Read the model definition and answer for the solid it produces. Units are mm, in the model's axes. Face numbers are marked on the shaded views. Coordinates: 2 decimals unless noted, no trailing zeros. Write each loop counter-clockwise with the first axis right and the second up, starting at its lowest first coordinate (ties: lowest second). Pieces come first, ordered by that corner, then holes.
(1) Straight lines are drawn through the part: line 1 along X through (y, z) = (0, -6.25); line 2 along Y through (x, z) = (0, 10.25). For each, find the intervals that lie inside material, in ascending order.
(2) The part is cut by section A-A, the plane x = 0. Determine the outline of the cut face in (y, z).
(3) The part is cut by section C-C, the plane z = 16.5. Determine the outline of the cut face in (x, y), and give its area (3 significant figures).
(4) Determine the mould class of the marked faces 1, 2 and 3 for opening direction X: pulls with the +X half, pulls with the -X half, needs draft (parallel to the pull), parting line crosses it, or undercut.
(5) Given pin 1 (5.5 mm diameter, centred on x = 0, y = 0, fed in from +Z); pin 2 (2 mm diameter, centred on y = -2.5, z = 9, fed in from +X); pin 3 (1.5 mm diameter, centred on x = 3, z = 17, fed in from +Y); pin 4 (1 mm diameter, centred on y = -1.5, z = 11.5, fed in from -X), each flat-ended and moving along its own axis, determine where each tip first touches the part or whether it passes through.
(6) The part is cut by section D-D, the plane z = -2. Determine the outline of the cut face in (x, y).
```python
from build123d import *

# Parameters (mm, degrees)
F0_R     = 6
F0_R_2   = 4
F1_DEPTH = 4
F2_DEPTH = 4
F3_R     = 6
F3_R_2   = 4.5
F4_DEPTH = 20
F5_R     = 6
F5_R_2   = 4.45
F6_DEPTH = 15
F7_SIZE  = 0.4
F8_R     = 1


with BuildPart() as f1:
    # F0 (on Top) → F1 (new body)
    with BuildSketch(Plane.XY):
        Circle(F0_R)
        Circle(F0_R_2, mode=Mode.SUBTRACT)
    extrude(amount=F1_DEPTH)

    # F0 (on Top) → F2 (join)
    with BuildSketch(Plane.XY):
        Circle(F0_R)
        Circle(F0_R_2, mode=Mode.SUBTRACT)
    extrude(amount=F2_DEPTH)

    # F3 (on face) → F4 (join)
    with BuildSketch(Plane.XY.offset(4)):
        Circle(F3_R)
        Circle(F3_R_2, mode=Mode.SUBTRACT)
    extrude(amount=F4_DEPTH)

    # F5 (on face) → F6 (join)
    with BuildSketch(Plane(origin=(0, 0, 0), x_dir=(1, 0, 0), z_dir=(0, 0, -1))):
        Circle(F5_R)
        Circle(F5_R_2, mode=Mode.SUBTRACT)
    extrude(amount=F6_DEPTH)

    # F7
    f7_edges = [f1.edges().sort_by_distance(p)[0] for p in [
        (-4.45, 0, -15),
        (-4.5, 0, 24),
    ]]
    chamfer(f7_edges, length=F7_SIZE)

    # F8
    f8_edges = [f1.edges().sort_by_distance(p)[0] for p in [
        (-6, 0, 24),
        (-6, 0, -15),
    ]]
    fillet(f8_edges, radius=F8_R)


solid = f1.part
```
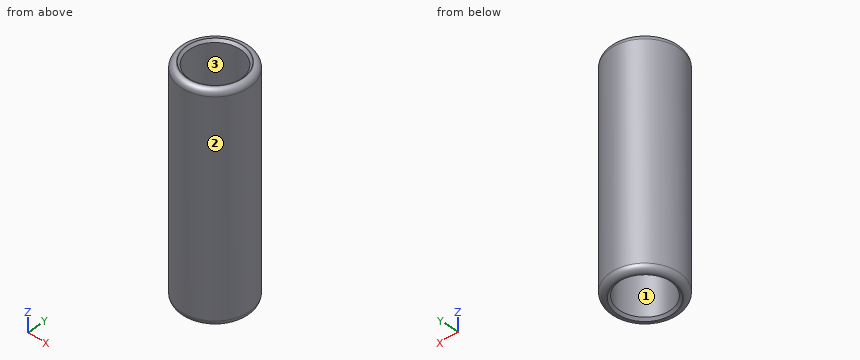
Computed:
1. line 1: x = -6 to -4.45, 4.45 to 6
1. line 2: y = -6 to -4.5, 4.5 to 6
2. outline: (-6, -14) arc R1 ccw to (-5, -15) - (-4.85, -15) - (-4.45, -14.6) - (-4.45, 0) - (-4, 0) - (-4, 4) - (-4.5, 4) - (-4.5, 23.6) - (-4.9, 24) - (-5, 24) arc R1 ccw to (-6, 23) - close; (4, 0) - (4.45, 0) - (4.45, -14.6) - (4.85, -15) - (5, -15) arc R1 ccw to (6, -14) - (6, 23) arc R1 ccw to (5, 24) - (4.9, 24) - (4.5, 23.6) - (4.5, 4) - (4, 4) - close
3. outline: circle Ø12 at (0, 0); hole circle Ø9 at (0, 0)
3. area: 49.5 mm2
4. face 1: undercut
4. face 2: parting line crosses it
4. face 3: undercut
5. pin 1: passes through
5. pin 2: stops at x = 5.81
5. pin 3: stops at y = 5.56
5. pin 4: stops at x = -5.92
6. outline: circle Ø12 at (0, 0); hole circle Ø8.9 at (0, 0)
